Autodesk Inventor part; units mm, degrees
ref_plane "YZ Plane" through (0, 0, 0) normal (1, 0, 0) x (0, 1, 0)
ref_plane "XZ Plane" through (0, 0, 0) normal (0, 1, 0) x (-1, 0, 0)
ref_plane "XY Plane" through (0, 0, 0) normal (0, 0, 1) x (1, 0, 0)
sketch "Sketch1" plane through (0, 0, 0) normal (0, 1, 0) x (-1, 0, 0)
  line L0 (-22.5, -6) -> (-22.5, 6)
  line L1 (-10.5, -6) -> (-5.8469, -1.3469)
  line L2 (-10.5, -6) -> (-3.9195, -6) construction
  line L3 (-10.5, 6) -> (-5.8469, 1.3469)
  arc A0 (-5.8469, -1.3469) -> (-5.8469, 1.3469) centre (-0.0057, 0) ccw
  line L4 (-22.5, 16) -> (-22.5, -16)
  line L5 (-22.5, -16) -> (-18.5, -16)
  line L6 (-18.5, 16) -> (-22.5, 16)
  line L7 (-18.5, -16) -> (-18.5, -6)
  line L8 (-18.5, 16) -> (-18.5, 6)
  line L9 (-10.5, 6) -> (-18.5, 6)
  line L10 (-10.5, -6) -> (-18.5, -6)
  point P0 (0, 0)
  dimension "d2" = 12
  dimension "d3" = 45
  dimension "d4" = 12
  dimension "d6" = 5.9944
  dimension "d7" = 32
  dimension "d8" = 4
  dimension "d10" = 0
extrude "Extrusion1" add sketch "Sketch1" along normal blind 750
properties part number "supportedRail_SBR12_750mm"
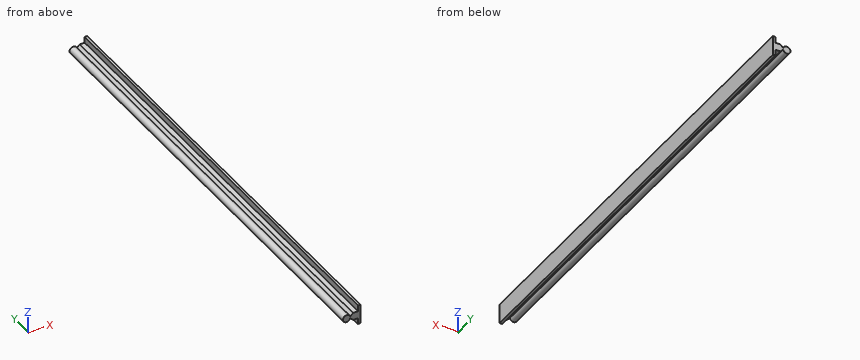
Read the model definition and answer for the solid it produces. Units are mm, in the model's axes. Round coordinates to 2 decimals unless told otherwise and drop trailing zeros. Write each loop counter-clockwise with the first axis right and the second up, starting at its lowest first coordinate (ties: lowest second). Pieces come first, ordered by that corner, then holes.
Q1. Straight lines are drawn through the part: line 1 (X direction, y = 570, z = 8); line 2 (X direction, y = 643, z = -5); line 3 (Z direction, x = 16.75, y = 266). For each, find the intervals that lie inside material, in ascending order.
Values:
line 1: x = 18.5 to 22.5
line 2: x = -3.3 to 3.31, 9.5 to 22.5
line 3: z = -6 to 6
Q2. Flat-ended cylindrical pins translate along their axes: P1, Ø1, axis at y = 646.5, z = 6, coming from the -X side; P2, Ø2, axis at x = 2, y = 603.5, coming from the -Z side; P3, Ø6.5, axis at x = 13.5, y = 459, coming from the -Z side. Find the tip coordinate at first contact, or state that the pin passes through.
Values:
P1: stops at x = -2.38
P2: stops at z = -5.91
P3: stops at z = -6
Q3. Find section A-A on y = 484.5. Determine the outline of the cut face in (x, z).
Values:
outline: (5.85, -1.35) - (10.5, -6) - (18.5, -6) - (18.5, -16) - (22.5, -16) - (22.5, 16) - (18.5, 16) - (18.5, 6) - (10.5, 6) - (5.85, 1.35) arc R5.99 ccw (long way) to start
Q4. Find section B-B on x = -0.75. Determine the outline of the cut face in (y, z), and give its area (3 significant figures).
Values:
outline: (0, -5.95) - (750, -5.95) - (750, 5.95) - (0, 5.95) - close
area: 8,920 mm2
